from build123d import *

# Parameters (mm, degrees)
SKETCH_1_R          = 30.428996358
SKETCH_1_R_2        = 16.155751461
EXTRUDE_2_DEPTH     = 24
SKETCH_2_R          = 62
CUT_EXTRUDE_1_DEPTH = 8


with BuildPart() as part:
    # Эскиз1 → Бобышка-Вытянуть2 (new body, symmetric)
    with BuildSketch(Plane(origin=(0, 0, 0), x_dir=(1, 0, 0), z_dir=(0, 1, 0))):
        with BuildLine():
            Line((6.227294987, 55.90193086), (114.792593034, 43.808106445))
            ThreePointArc((114.792593034, 43.808106445), (153.990225093, -0.347161193), (114.101954958, -43.879539083))
            Line((114.101954958, -43.879539083), (-4.795118465, -56.042947064))
            ThreePointArc((-4.795118465, -56.042947064), (-55.977019444, 5.511657733), (6.227294987, 55.90193086))
        make_face()
        Circle(SKETCH_1_R, mode=Mode.SUBTRACT)
        with Locations((109.912511122, 0)):
            Circle(SKETCH_1_R_2, mode=Mode.SUBTRACT)
    extrude(amount=EXTRUDE_2_DEPTH, both=True)

    # Эскиз2 → Вырез-Вытянуть1 (cut, symmetric)
    with BuildSketch(Plane(origin=(0, 0, 0), x_dir=(1, 0, 0), z_dir=(0, 1, 0))):
        with Locations((109.912511122, 0)):
            Circle(SKETCH_2_R)
    extrude(amount=CUT_EXTRUDE_1_DEPTH, both=True, mode=Mode.SUBTRACT)


solid = part.part
Geometry: final body of the model. Coordinates: model frame, mm. A direction names the side the tool comes from. Give positions to 0.01 mm unless a question says otherwise; leave off trailing zeros. Order: outer loops, then holes, each group sorted by start corner. A loop starts at its lowest first (then second) coordinate and runs counter-clockwise, first axis right, second up. Notation, with made-up numbers: (78, 82.5) -> (106, 82.5) arc R17 cw to (106, 86.5) -> close; hole circle Ø9 at (-17, 73). An arc over 180 degrees is marked (long way). Write each question's results on one line, items separated by ' | '.
1) Line query: line 1 along X through (y, z) = (18, 0); line 2 along Y through (x, z) = (126, 20.5); line 3 along X through (y, z) = (5.5, 0). Output: solid intervals per line, ascending.
Geometry says:
line 1: x = -56.25 to -30.43, 30.43 to 93.76, 126.07 to 153.99 | line 2: y = -24 to -8, 8 to 24 | line 3: x = -56.25 to -30.43, 30.43 to 47.91
2) Cut plane C-C (x = 0). Output: boundary loops of the cut face in (y, z).
Geometry says:
outline: (-24, -56.25) -> (24, -56.25) -> (24, -30.43) -> (-24, -30.43) -> close; (-24, 30.43) -> (24, 30.43) -> (24, 55.55) -> (-24, 55.55) -> close
3) Cut plane A-A (z = 0). Output: boundary loops of the cut face in (x, y), and give its area (3 significant figures).
Geometry says:
outline: (-56.25, -24) -> (-30.43, -24) -> (-30.43, 24) -> (-56.25, 24) -> close; (30.43, -24) -> (93.76, -24) -> (93.76, -8) -> (47.91, -8) -> (47.91, 8) -> (93.76, 8) -> (93.76, 24) -> (30.43, 24) -> close; (126.07, -24) -> (153.99, -24) -> (153.99, -8) -> (126.07, -8) -> close; (126.07, 8) -> (153.99, 8) -> (153.99, 24) -> (126.07, 24) -> close | area: 4,440 mm²
4) Draft query along X for faces 3 (the face through (124.836, 15.888, 6.188)), 4 (the face through (-22.427, -0.336, -20.565)), 5 (the face through (50, -24, -1)), 6 (the face through (59.75, 0.34, -49.94)). Return one class per face: released by +X, released by -X, zero draft, split by the parting line, or undercut.
Geometry says:
face 3: undercut | face 4: undercut | face 5: zero draft | face 6: released by +X
5) First-contact query: pin 1 Ø5 at (x, y) = (44, -9.5) entering from +Z; pin 2 Ø5 at (y, z) = (19, -39) entering from +X; pin 3 Ø1.5 at (y, z) = (-7, 30.5) entering from -X; pin 4 Ø12 at (x, z) = (-20.5, -12) entering from +Y (3 decimals). Flat tips, straight axial feed; report the tip coordinate or a pass-through.
Geometry says:
pin 1: stops at z = 51.31 | pin 2: stops at x = 134.63 | pin 3: stops at x = -47.74 | pin 4: passes through
6) Set-up query: faces 1 (the face through (124.836, -16.112, 6.188)), 2 (the face through (47.92, 0.11, -1.06)). Return all of +Z, -Z, +X, -X, +Y, -Y with unobstructed straight access to the full face (end or side cutting, diameter ignored); none if empty.
Geometry says:
face 1: +Y, -Y | face 2: +X
7) Cut plane B-B (y = -19). Output: boundary loops of the cut face in (x, z), and give its area (3 significant figures).
Geometry says:
outline: (-4.8, 56.04) arc R56.25 ccw (long way) to (6.23, -55.9) -> (114.79, -43.81) arc R44.08 ccw to (114.1, 43.88) -> close; hole circle Ø60.86 at (0, 0); hole circle Ø32.31 at (109.91, 0) | area: 15,300 mm²
8) Cut plane D-D (x = 104). Output: boundary loops of the cut face in (y, z), and give its area (3 significant figures).
Geometry says:
outline: (-24, -45.01) -> (-8, -45.01) -> (-8, -15.03) -> (-24, -15.03) -> close; (-24, 15.03) -> (-8, 15.03) -> (-8, 44.91) -> (-24, 44.91) -> close; (8, -45.01) -> (24, -45.01) -> (24, -15.03) -> (8, -15.03) -> close; (8, 15.03) -> (24, 15.03) -> (24, 44.91) -> (8, 44.91) -> close | area: 1,920 mm²
